Read the model definition and answer for the solid it produces. Units are mm, in the model's axes. Give positions to 0.01 mm unless a question says otherwise; leave off trailing zeros. Order: outer loops, then holes, each group sorted by start corner. A loop starts at its lowest first (then second) coordinate and runs counter-clockwise, first axis right, second up. Notation, with made-up numbers: (65.5, 17) -> (88.5, 17) arc R20 ccw to (88.5, 24) -> close; hole circle Ø10 at (-6, -36). An arc over 180 degrees is marked (long way). Answer as CSV lines item,"result". Start each with the question number.
1) Find section C-C (x = -15.5). Determine the outline of the cut face in (y, z), and give its area (3 significant figures).
2) Find section B-B (z = -41). Determine the outline of the cut face in (x, y), and give its area (3 significant figures).
3) Find section A-A (x = 0). Determine the outline of the cut face in (y, z).
4) Straight lines are drawn through the part: L1, parallel to X at y = 1.7, z = -12.5; L2, parallel to Z at x = -4, y = 5.1; L3, parallel to Z at x = -9, y = 0.45. For each, find the intervals that lie inside material, in ascending order. Write a range as from..to.
5) Find section D-D (y = 3.9). State how many separate pieces and enclosed holes the cut face has, and give its area (3 significant figures).
6) Flat-ended cylindrical pins translate along their axes: pin 1 Ø1 at (y, z) = (1, -36) entering from +X; pin 2 Ø2 at (x, y) = (30, 3) entering from +Z. Find the tip coordinate at first contact, or state that the pin passes through.
Autodesk Inventor part; units mm, degrees
ref_plane "YZ Plane" through (0, 0, 0) normal (1, 0, 0) x (0, 1, 0)
ref_plane "XZ Plane" through (0, 0, 0) normal (0, 1, 0) x (-1, 0, 0)
ref_plane "XY Plane" through (0, 0, 0) normal (0, 0, 1) x (1, 0, 0)
sketch "Sketch1" plane through (0, 0, 0) normal (0, 1, 0) x (-1, 0, 0)
  line L0 (-55, -52.5) -> (-24.8972, 11.6781)
  line L1 (-55, -82.5) -> (-55, -52.5)
  line L2 (27.5, 0) -> (27.5, -82.5)
  line L3 (9.5, -64.5) -> (-37, -64.5)
  line L4 (9.5, -64.5) -> (9.5, -25.807)
  line L5 (-37, -64.5) -> (-37, -56.5118)
  arc A0 (27.5, 0) -> (-24.8972, 11.6781) centre (0, 0) ccw
  arc A1 (-19.56, -19.3302) -> (9.5, -25.807) centre (0, 0) ccw
  circle A2 centre (0, 7) radius 6.25
  circle A3 centre (15.5, 0) radius 1.6
  circle A4 centre (7.75, 13.4234) radius 1.6
  circle A5 centre (-7.75, 13.4234) radius 1.6
  circle A6 centre (-15.5, 0) radius 1.6
  circle A7 centre (-7.75, -13.4234) radius 1.6
  circle A8 centre (7.75, -13.4234) radius 1.6
  line L6 (-19.56, -19.3302) -> (-37, -56.5118)
  line L7 (27.5, -82.5) -> (-55, -82.5)
  dimension "d12" = 18
  dimension "d13" = 82.5
  dimension "d14" = 12.5
  dimension "d15" = 7
  dimension "d16" = 3.2
  dimension "d17" = 15.5
  dimension "d20" = 360
  dimension "d22" = 30
  dimension "d23" = 27.5
  dimension "d24" = 18
  dimension "d25" = 27.5
  dimension "d26" = 27.5
  dimension "d27" = 27.5
  dimension "d29" = 18
  dimension "d30" = 18
  dimension "d31" = 82.5
  dimension "d32" = 82.5
extrude "Extrusion1" add sketch "Sketch1" along normal blind 6
properties part number "chassi_front_template"
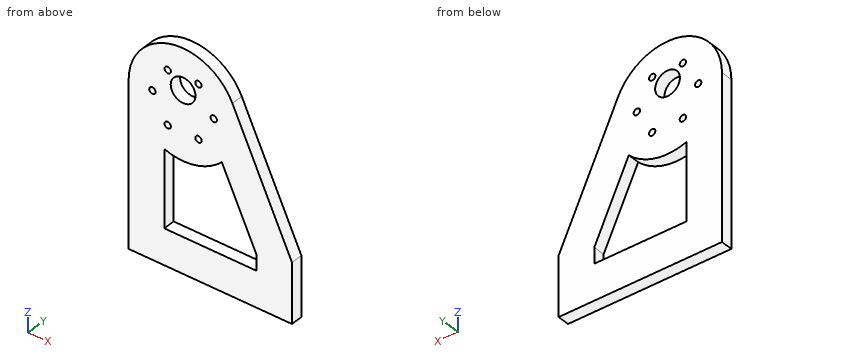
Findings below:
1,outline,"(0, -82.5) -> (6, -82.5) -> (6, -1.6) -> (0, -1.6) -> close; (0, 1.6) -> (6, 1.6) -> (6, 22.72) -> (0, 22.72) -> close"
1,area,"612 mm²"
2,outline,"(-27.5, 0) -> (-9.5, 0) -> (-9.5, 6) -> (-27.5, 6) -> close; (29.72, 0) -> (49.61, 0) -> (49.61, 6) -> (29.72, 6) -> close"
2,area,"227 mm²"
3,outline,"(0, -82.5) -> (6, -82.5) -> (6, -64.5) -> (0, -64.5) -> close; (0, -27.5) -> (6, -27.5) -> (6, 0.75) -> (0, 0.75) -> close; (0, 13.25) -> (6, 13.25) -> (6, 27.5) -> (0, 27.5) -> close"
4,L1,"-27.5..-9.06, -6.44..6.44, 9.06..36.24"
4,L2,"-82.5..-64.5, -27.21..2.2, 11.8..27.21"
4,L3,"-82.5..-64.5, -25.99..-14.42, -12.42..12.42, 14.42..25.99"
5,separate pieces,"1"
5,enclosed holes,"8"
5,area,"5,590 mm²"
6,pin 1,"x = 47.5"
6,pin 2,"z = 2.93"
